Check sheet for the modelled part. Datum: model origin and axes. Units: mm. A direction names the side the tool comes from. Give positions to 0.01 mm unless a question says otherwise; leave off trailing zeros. Order: outer loops, then holes, each group sorted by start corner. A loop starts at its lowest first (then second) coordinate and runs counter-clockwise, first axis right, second up. Notation, with made-up numbers: (87.25, -29) -> (141.25, -29) arc R15 cw to (141.25, -22) -> close; hole circle Ø8 at (40, -2.75). An arc over 180 degrees is marked (long way). Write each question's results on one line, items separated by ' | '.
from build123d import *

# Parameters (mm, degrees)
SKETCH2_W                                = 80
SKETCH2_H                                = 80
BOSS_EXTRUDE1_DEPTH                      = 85
SKETCH3_W                                = 30
SKETCH3_H                                = 40
CUT_EXTRUDE1_DEPTH                       = 124.389626793
SKETCH4_R                                = 15
BOSS_EXTRUDE2_DEPTH                      = 20
SKETCH5_R                                = 15
BOSS_EXTRUDE3_DEPTH                      = 5
SKETCH7_R                                = 30
BOSS_EXTRUDE4_DEPTH                      = 45
BOSS_EXTRUDE5_DEPTH                      = 30
CUT_EXTRUDE2_DEPTH                       = 15
SKETCH11_W                               = 60
SKETCH11_H                               = 60
CUT_EXTRUDE3_DEPTH                       = 75
BOSS_EXTRUDE6_DEPTH                      = 30
SKETCH21_R                               = 15
BOSS_EXTRUDE7_DEPTH                      = 10
F_20_0_20_DIAMETER_HOLE1_D               = 20
F_20_0_20_DIAMETER_HOLE2_D               = 20
F_20_0_20_DIAMETER_HOLE3_D               = 20
CBORE_FOR_M10_HEX_HEAD_BOLT2_D           = 10
CBORE_FOR_M10_HEX_HEAD_BOLT2_CBORE_D     = 20
CBORE_FOR_M10_HEX_HEAD_BOLT2_CBORE_DEPTH = 15
BOSS_EXTRUDE9_DEPTH                      = 5
SKETCH25_W                               = 10
SKETCH25_H                               = 10
CUT_EXTRUDE4_DEPTH                       = 60
FILLET1_R                                = 10


with BuildPart() as part:
    # Sketch2 → Boss-Extrude1 (new body)
    with BuildSketch(Plane(origin=(0, 0, 0), x_dir=(1, 0, 0), z_dir=(0, 1, 0))):
        Rectangle(SKETCH2_W, SKETCH2_H)
    extrude(amount=BOSS_EXTRUDE1_DEPTH)

    # Sketch3 → Cut-Extrude1 (cut, through all)
    with BuildSketch(Plane.XY.offset(40)):
        Rectangle(SKETCH3_W, SKETCH3_H)
    extrude(amount=-CUT_EXTRUDE1_DEPTH, mode=Mode.SUBTRACT)

    # Sketch4 → Boss-Extrude2 (add)
    with BuildSketch(Plane(origin=(0, 0, -40), x_dir=(-1, 0, 0), z_dir=(0, 0, -1))):
        with Locations((0, 55)):
            Circle(SKETCH4_R)
    extrude(amount=BOSS_EXTRUDE2_DEPTH)

    # Sketch5 → Boss-Extrude3 (add)
    with BuildSketch(Plane(origin=(0, 85, 0), x_dir=(1, 0, 0), z_dir=(0, 1, 0))):
        with Locations(Location((0, 0, 0), (0, 0, 270))):
            Circle(SKETCH5_R)
    extrude(amount=BOSS_EXTRUDE3_DEPTH)



with BuildPart() as body_2:
    # Sketch7 → Boss-Extrude4 (new body)
    with BuildSketch(Plane(origin=(0, 0, 0), x_dir=(1, 0, 0), z_dir=(0, 1, 0))):
        with Locations(Location((-100, 0, 0), (0, 0, 90))):
            Circle(SKETCH7_R)
    extrude(amount=BOSS_EXTRUDE4_DEPTH)


with BuildPart() as part_1:
    add(part.part)

    add(body_2.part)  # Boss-Extrude5 merges body 2
    # Sketch9 → Boss-Extrude5 (add)
    with BuildSketch(Plane(origin=(0, 0, 0), x_dir=(1, 0, 0), z_dir=(0, 1, 0))):
        with BuildLine():
            Line((-40, 0), (-40, 40))
            Line((-40, 40), (-104.747935056, 29.621902584))
            ThreePointArc((-104.747935056, 29.621902584), (-80.53770378, 22.830221765), (-70, 0))
            Line((-70, 0), (-40, 0))
        make_face()
        with BuildLine():
            Line((-40, -40), (-40, 0))
            Line((-40, 0), (-70, 0))
            ThreePointArc((-70, 0), (-80.53770378, -22.830221765), (-104.747935056, -29.621902584))
            Line((-104.747935056, -29.621902584), (-40, -40))
        make_face()
    extrude(amount=BOSS_EXTRUDE5_DEPTH)

    # Sketch10 → Cut-Extrude2 (cut)
    with BuildSketch(Plane.XZ):
        with BuildLine():
            Line((-50, 28.269512751), (-103.165290037, 19.747935056))
            ThreePointArc((-103.165290037, 19.747935056), (-120, 0), (-103.165290037, -19.747935056))
            Line((-103.165290037, -19.747935056), (-50, -28.269512751))
            Line((-50, -28.269512751), (-50, 28.269512751))
        make_face()
    extrude(amount=-CUT_EXTRUDE2_DEPTH, mode=Mode.SUBTRACT)

    # Sketch11 → Cut-Extrude3 (cut)
    with BuildSketch(Plane.XZ):
        Rectangle(SKETCH11_W, SKETCH11_H)
    extrude(amount=-CUT_EXTRUDE3_DEPTH, mode=Mode.SUBTRACT)

    # Sketch12 → Boss-Extrude6 (add)
    with BuildSketch(Plane(origin=(0, 0, 0), x_dir=(1, 0, 0), z_dir=(0, 1, 0))):
        with BuildLine():
            Line((40, 30), (78.377223398, 30))
            ThreePointArc((78.377223398, 30), (86.395060656, 32.322686179), (91.929841942, 38.571428571))
            ThreePointArc((91.929841942, 38.571428571), (114.392996633, 49.511575554), (130, 30))
            Line((130, 30), (130, -30))
            ThreePointArc((130, -30), (114.392996633, -49.511575554), (91.929841942, -38.571428571))
            ThreePointArc((91.929841942, -38.571428571), (86.395060656, -32.322686179), (78.377223398, -30))
            Line((78.377223398, -30), (40, -30))
            Line((40, -30), (40, 30))
        make_face()
    extrude(amount=BOSS_EXTRUDE6_DEPTH)

    # Sketch21 → Boss-Extrude7 (add)
    with BuildSketch(Plane(origin=(0, 30, 0), x_dir=(1, 0, 0), z_dir=(0, 1, 0))):
        with Locations(Location((110, 30, 0), (0, 0, 90))):
            Circle(SKETCH21_R)
        with Locations(Location((110, -30, 0), (0, 0, 90))):
            Circle(SKETCH21_R)
    extrude(amount=BOSS_EXTRUDE7_DEPTH)

    # Ø20.0 (20) Diameter Hole1 (through all)
    with Locations(Plane(origin=(0, 45, 0), x_dir=(1, 0, 0), z_dir=(0, 1, 0))):
        with Locations((-100, 0)):
            Hole(F_20_0_20_DIAMETER_HOLE1_D / 2)

    # Ø20.0 (20) Diameter Hole2 (through all)
    with Locations(Plane(origin=(0, 90, 0), x_dir=(1, 0, 0), z_dir=(0, 1, 0))):
        with Locations((0, 0)):
            Hole(F_20_0_20_DIAMETER_HOLE2_D / 2)

    # Ø20.0 (20) Diameter Hole3 (through all)
    with Locations(Plane(origin=(0, 0, -60), x_dir=(-1, 0, 0), z_dir=(0, 0, -1))):
        with Locations((0, 55)):
            Hole(F_20_0_20_DIAMETER_HOLE3_D / 2)

    # CBORE for M10 Hex Head Bolt2 (through all)
    with Locations(Plane(origin=(0, 40, 0), x_dir=(1, 0, 0), z_dir=(0, 1, 0))):
        with Locations((110, 30), (110, -30)):
            CounterBoreHole(CBORE_FOR_M10_HEX_HEAD_BOLT2_D / 2, CBORE_FOR_M10_HEX_HEAD_BOLT2_CBORE_D / 2, CBORE_FOR_M10_HEX_HEAD_BOLT2_CBORE_DEPTH)

    # Sketch24 → Boss-Extrude9 (add, symmetric)
    with BuildSketch(Plane.XY):
        Polygon((-40, 85), (-70, 45), (-71.999098595, 45), (-71.999098595, 30), (-70, 30), (-40, 30), align=None)
    extrude(amount=BOSS_EXTRUDE9_DEPTH, both=True)

    # Sketch25 → Cut-Extrude4 (cut)
    with BuildSketch(Plane(origin=(130, 0, 0), x_dir=(0, 0, -1), z_dir=(1, 0, 0))):
        with Locations((0, 25)):
            Rectangle(SKETCH25_W, SKETCH25_H)
    extrude(amount=-CUT_EXTRUDE4_DEPTH, mode=Mode.SUBTRACT)

    # Fillet1
    fillet1_edges = [part_1.edges().sort_by_distance(p)[0] for p in [
        (-30, 37.5, 30),
        (30, 37.5, -30),
        (-30, 37.5, -30),
        (30, 37.5, 30),
    ]]
    fillet(fillet1_edges, radius=FILLET1_R)


solid = part_1.part
1. Section check D-D on x = 0. Record the cut outline in (y, z).
Verdict:
outline: (20, -40) -> (40, -40) -> (40, -60) -> (45, -60) -> (45, -30) -> (20, -30) -> close; (20, 30) -> (45, 30) -> (45, 40) -> (20, 40) -> close; (65, -60) -> (70, -60) -> (70, -40) -> (85, -40) -> (85, -15) -> (90, -15) -> (90, -10) -> (75, -10) -> (75, -30) -> (65, -30) -> close; (65, 30) -> (75, 30) -> (75, 10) -> (90, 10) -> (90, 15) -> (85, 15) -> (85, 40) -> (65, 40) -> close
2. Section check B-B on y = 55. Record the cut outline in (x, z).
Verdict:
outline: (-62.5, -5) -> (-40, -5) -> (-40, -40) -> (-15, -40) -> (-15, -60) -> (-10, -60) -> (-10, -30) -> (-20, -30) arc R10 cw to (-30, -20) -> (-30, 20) arc R10 cw to (-20, 30) -> (-10, 30) -> (-10, 40) -> (-40, 40) -> (-40, 5) -> (-62.5, 5) -> close; (10, -60) -> (15, -60) -> (15, -40) -> (40, -40) -> (40, 40) -> (10, 40) -> (10, 30) -> (20, 30) arc R10 cw to (30, 20) -> (30, -20) arc R10 cw to (20, -30) -> (10, -30) -> close
3. Mould release check, pull along Z, two halves, no side actions. Record for faces 6 (the flat face through (30, 37, 0)), 7 (the cylindrical face through (0.66, 87.465, -14.985)), 8 (the flat face through (-40, 57, 23)): +Z half, -Z half, draft (parallel to the pull), parting line (faces both ways), or undercut.
Verdict:
face 6: undercut | face 7: parting line | face 8: draft
4. Section check A-A on x = 110. Give the number of separate pieces and of enclosed holes in the cut face, then the cut area to 3 significant figures.
Verdict:
separate pieces: 3 | enclosed holes: 0 | area: 2,400 mm^2
5. Gauge pin test, flat ends, axial feed: pin 1 Ø4.5 at (y, z) = (4, -10) entering from -X; pin 2 Ø5 at (x, z) = (78, 0.5) entering from +Y; pin 3 Ø15 at (x, z) = (106.5, 35) entering from +Y; pin 4 Ø9 at (x, y) = (-62, 68) entering from +Z. Record the tip position at first contact, or that the pin passes through.
Verdict:
pin 1: stops at x = -128.98 | pin 2: stops at y = 20 | pin 3: stops at y = 40 | pin 4: passes through
6. Access from +Z, -Z, +X, -X, +Y, -Y to the whole of each face (thin tool, end or side, straight path). Record for faces 1 (the flat face through (15, 10, -35)), 2 (the flat face through (59, 15, 30)), 3 (the flat face through (59, 15, -30)), 4 (the flat face through (-30, 37, 0)), 5 (the cylindrical face through (109.34, 34.93, 44.985)).
Verdict:
face 1: +Z, -Z, -Y | face 2: +Z, +Y, -Y | face 3: -Z, +Y, -Y | face 4: -Y | face 5: +Y
7. Material ranges on probe 1 along Z at (x, y) = (110, 7); probe 2 along Z at (x, y) = (110, 34); probe 3 along X at (y, z) = (59.5, 18.5), recorded low to high. Write a range as from..to.
Verdict:
probe 1: z = -50..-35, -25..25, 35..50 | probe 2: z = -45..-40, -20..-15, 15..20, 40..45 | probe 3: x = -40..-30, 30..40
